```python
from build123d import *

# Parameters (mm, degrees)
SKETCH1_R           = 5
BOSS_EXTRUDE1_DEPTH = 10


# Read off the part's stored shape, not the designer's step: Imported1
with BuildPart() as part:
    # Sketch1 → Boss-Extrude1 (new body)
    with BuildSketch(Plane(origin=(0, 0, 0), x_dir=(1, 0, 0), z_dir=(0, 1, 0))):
        with BuildLine():
            Line((-30, 40), (25, 40))
            Line((25, 40), (30.478825766, 30.510395408))
            Line((30.478825766, 30.510395408), (21.818571728, 25.510395408))
            Line((21.818571728, 25.510395408), (31.818571728, 8.189887333))
            Line((31.818571728, 8.189887333), (40.478825766, 13.189887333))
            Line((40.478825766, 13.189887333), (50.478825766, -4.130620743))
            Line((50.478825766, -4.130620743), (41.818571728, -9.130620743))
            Line((41.818571728, -9.130620743), (51.818571728, -26.451128819))
            Line((51.818571728, -26.451128819), (60.478825766, -21.451128819))
            Line((60.478825766, -21.451128819), (69.659283069, -37.352147305))
            Line((69.659283069, -37.352147305), (21.766908157, -41.979610283))
            Line((21.766908157, -41.979610283), (19.644977926, -35.595148029))
            Line((19.644977926, -35.595148029), (17.593976856, -29.424097387))
            ThreePointArc((17.593976856, -29.424097387), (14.880225334, -25.223606168), (10.471929596, -22.862355971))
            Line((10.471929596, -22.862355971), (-0.170430849, -20.268984513))
            ThreePointArc((-0.170430849, -20.268984513), (-10.525131482, -22.513169462), (-15.157047212, -32.042154085))
            Line((-15.157047212, -32.042154085), (-15.157047212, -56.665547585))
            Line((-15.157047212, -56.665547585), (-50, -57.51739948))
            Line((-50, -57.51739948), (-50, -33.474160509))
            Line((-50, -33.474160509), (-50, 20))
            ThreePointArc((-50, 20), (-44.142135624, 34.142135624), (-30, 40))
        make_face()
        with Locations(Location((0, 0, 0), (0, 0, 90))):
            Circle(SKETCH1_R, mode=Mode.SUBTRACT)
    extrude(amount=BOSS_EXTRUDE1_DEPTH)


solid = part.part
```
The listing builds one solid part. Answer for the finished solid, in the listing's coordinates (mm). A direction names the side the tool comes from. Coordinates: 2 decimals unless noted, no trailing zeros. Loops run counter-clockwise (first coordinate to the right, second up) from the corner with the lowest first, then second, coordinate; pieces in that order, holes last. Notation, with made-up numbers: M -31,5 L 17,5 A6 cw 17,16 Z; hole C -36,68 d7. An arc over 180 degrees is marked long. Answer as CSV lines item,"result". Start each with the question number.
(1) The part is cut by section B-B (z = 0). Give the vertices of the cut face in (x, y), and give its area (3 significant figures).
(2) The part is cut by section D-D (z = -10.5). Give the vertices of the cut face in (x, y), and give its area (3 significant figures).
(3) Given pin 1 (1 mm diameter, centred on y = 3.5, z = -7, fed in from +X); pin 2 (6 mm diameter, centred on x = 6.5, y = 7, fed in from +Z); pin 3 (4 mm diameter, centred on y = 3, z = -29, fed in from -X) (3 decimals), each flat-ended and moving along its own axis, determine where each tip first touches the part or whether it passes through.
(4) The part is cut by section C-C (x = 56). Give the vertices of the cut face in (y, z).
(5) The mould has two halves that part along Z. Classify faces 4 (the cylindrical face through (4.88, 4.93, 1.08)), 5 (the cylindrical face through (-44.297, 4.93, -33.986)), 6 (the flat face through (26.209, 4.93, -28.045)), 7 (the flat face through (5.225, 4.93, 21.584)): pulls with the +Z half, pulls with the -Z half, needs draft (parallel to the pull), parting line crosses it, or undercut.
(6) Find the intervals of material crossed by L1, parallel to X at y = 3.75, z = 24; L2, parallel to Z at x = 50, y = 9; L3, parallel to Z at x = 23.5, y = 8.5, in increasing order. Write a range as [from, to].
(7) The part is cut by section A-A (y = 8.5). Give the vertices of the cut face in (x, z).
(8) For faces 1 (the flat face through (19.71, 4.93, 35.79)), 2 (the flat face through (46.2, 4.9, 6.6)), 3 (the flat face through (56.088, 4.93, 23.986)), determine the directions among +Z, -Z, +X, -X, +Y, -Y from which every point of the face is accessible in a straight line to the end or side of a thin tool.
Determined:
1,outline,"M -50,0 L -5,0 L -5,10 L -50,10 Z; M 5,0 L 48.09,0 L 48.09,10 L 5,10 Z"
1,area,"881 mm2"
2,outline,"M -50,0 L 30.48,0 L 30.48,10 L -50,10 Z; M 35.82,0 L 42.03,0 L 42.03,10 L 35.82,10 Z"
2,area,"867 mm2"
3,pin 1,"x = 44.34"
3,pin 2,"z = 22.63"
3,pin 3,"x = -48.735"
4,outline,"M 0,24.04 L 10,24.04 L 10,38.67 L 0,38.67 Z"
5,face 4,"undercut"
5,face 5,"pulls with the -Z half"
5,face 6,"undercut"
5,face 7,"pulls with the +Z half"
6,L1,"[-50, -12.1], [13.24, 50.4], [56.06, 61.95]"
6,L2,"[3.3, 4.41], [23.3, 39.25]"
6,L3,"[-40, -26.48], [-22.6, 41.81]"
7,outline,"M -50,-20 A20 ccw -30,-40 L 25,-40 L 30.48,-30.51 L 21.82,-25.51 L 31.82,-8.19 L 40.48,-13.19 L 50.48,4.13 L 41.82,9.13 L 51.82,26.45 L 60.48,21.45 L 69.66,37.35 L 21.77,41.98 L 17.59,29.42 A10 cw 10.47,22.86 L -0.17,20.27 A12.12 cw -15.16,32.04 L -15.16,56.67 L -50,57.52 Z; hole C 0,0 d10"
8,face 1,"+Z, +Y, -Y"
8,face 2,"+X, +Y, -Y"
8,face 3,"-Z, +Y, -Y"
